Input: part model. Units: mm. Frame: model coordinates. Give positions to 0.01 mm unless a question says otherwise; leave off trailing zeros. Write each loop counter-clockwise with the first axis right and the second up, starting at its lowest first coordinate (ties: lowest second). Pieces come first, ordered by that corner, then holes.
```python
from build123d import *

# Parameters (mm, degrees)
SKETCH1_W           = 60
SKETCH1_H           = 40
BOSS_EXTRUDE1_DEPTH = 2
SKETCH2_W           = 57
SKETCH2_H           = 37
BOSS_EXTRUDE2_DEPTH = 2
FILLET1_R           = 1
FILLET2_R           = 1


with BuildPart() as part:
    # Sketch1 → Boss-Extrude1 (new body)
    with BuildSketch(Plane(origin=(0, 0, 0), x_dir=(1, 0, 0), z_dir=(0, 1, 0))):
        Rectangle(SKETCH1_W, SKETCH1_H)
    extrude(amount=BOSS_EXTRUDE1_DEPTH)

    # Sketch2 → Boss-Extrude2 (add)
    with BuildSketch(Plane(origin=(0, 0, 0), x_dir=(1, 0, 0), z_dir=(0, 1, 0))):
        Rectangle(SKETCH2_W, SKETCH2_H)
    extrude(amount=-BOSS_EXTRUDE2_DEPTH)

    # Fillet1
    fillet1_edges = [part.edges().sort_by_distance(p)[0] for p in [
        (-30, 2, 0),
        (0, 2, 20),
        (30, 2, 0),
        (0, 2, -20),
    ]]
    fillet(fillet1_edges, radius=FILLET1_R)

    # Fillet2
    fillet2_edges = [part.edges().sort_by_distance(p)[0] for p in [
        (28.5, -2, 0),
        (0, -2, 18.5),
        (-28.5, -2, 0),
        (0, -2, -18.5),
    ]]
    fillet(fillet2_edges, radius=FILLET2_R)


solid = part.part
```
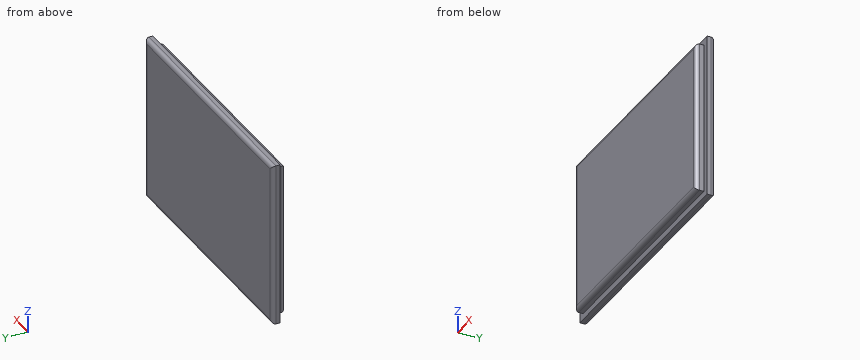
Item 1: Pin query (flat end, axial travel): pin 1 (0.5 mm diameter, centred on y = -0.5, z = -7.5, fed in from +X); pin 2 (0.8 mm diameter, centred on y = -0.5, z = -6.5, fed in from -X). Return the tip coordinate at first contact, or that it passes through.
Item 2: Section A-A (x = -2.5). Return loops of the section in (y, z), and give its area (3 significant figures).
Item 3: Section B-B (z = 7). Return loops of the section in (x, y), and give its area (3 significant figures).
Item 4: Ray query, line 1 (X direction, y = -0.8, z = -11); line 2 (Z direction, x = -17, y = -0.65); line 3 (X direction, y = 1.15, z = 11). Return the intervals inside material, ascending.
Solved:
1. pin 1: stops at x = 28.5
1. pin 2: stops at x = -28.5
2. outline: (-2, -17.5) arc R1 ccw to (-1, -18.5) - (0, -18.5) - (0, -20) - (1, -20) arc R1 ccw to (2, -19) - (2, 19) arc R1 ccw to (1, 20) - (0, 20) - (0, 18.5) - (-1, 18.5) arc R1 ccw to (-2, 17.5) - close
2. area: 153 mm2
3. outline: (-30, 0) - (-28.5, 0) - (-28.5, -1) arc R1 ccw to (-27.5, -2) - (27.5, -2) arc R1 ccw to (28.5, -1) - (28.5, 0) - (30, 0) - (30, 1) arc R1 ccw to (29, 2) - (-29, 2) arc R1 ccw to (-30, 1) - close
3. area: 233 mm2
4. line 1: x = -28.5 to 28.5
4. line 2: z = -18.5 to 18.5
4. line 3: x = -29.99 to 29.99
